For this review, take the finished solid that the model builds, in its own axes (mm). Round coordinates to 2 decimals unless told otherwise and drop trailing zeros. Write each loop counter-clockwise with the first axis right and the second up, starting at its lowest first coordinate (ties: lowest second). Pieces come first, ordered by that corner, then holes. Notation, with made-up numbers: (79.25, 54) -> (100.25, 54) arc R12 cw to (100.25, 58) -> close; hole circle Ø3 at (-5.5, -13). An arc over 180 degrees is marked (long way). Answer as CSV lines item,"result". Start each with the question number.
Item 1: Take a section at A-A on y = 96.5. Give the boundary of the cut face in (x, z).
Item 2: Wall thickness on probe 1 along Y at (x, z) = (1.6, -1.6); probe 2 along X at (y, z) = (72.5, 0): over which ranges is each line inside the solid? List them lowest first. Write a range as from..to.
Item 3: For pin 1 Ø1 at (y, z) = (43.5, 0.5) entering from -X; pin 2 Ø3.5 at (x, z) = (0, 0) entering from -Y; pin 3 Ø0.5 at (y, z) = (3, -2.5) entering from +X, all flat-tipped, find the tip position at first contact; note any pin that passes through.
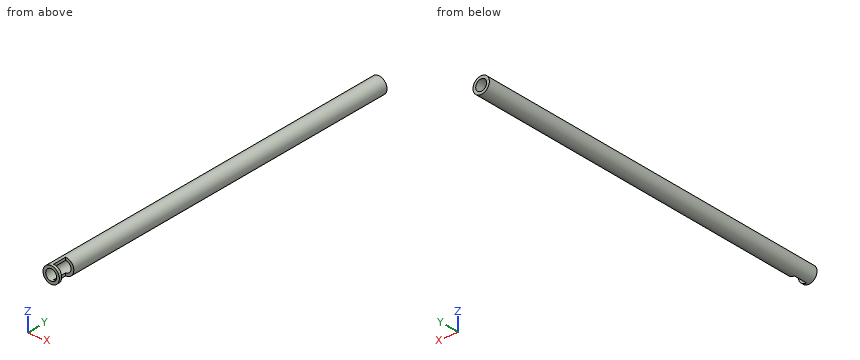
Autodesk Inventor part; units mm, degrees
ref_plane "YZ Plane" through (0, 0, 0) normal (1, 0, 0) x (0, 1, 0)
ref_plane "XZ Plane" through (0, 0, 0) normal (0, 1, 0) x (-1, 0, 0)
ref_plane "XY Plane" through (0, 0, 0) normal (0, 0, 1) x (1, 0, 0)
sketch "Szkic1" plane through (0, 0, 0) normal (0, 1, 0) x (-1, 0, 0)
  circle A0 centre (0, 0) radius 3
  circle A1 centre (0, 0) radius 2
  dimension "d0" = 6
  dimension "d1" = 4
extrude "Wyciągnięcie proste1" add sketch "Szkic1" along normal blind 135
sketch "Szkic2" plane through (0, 0, 0) normal (0, -1, 0) x (1, 0, 0)
  circle A0 centre (0, 0) radius 2
  circle A1 centre (0, 0) radius 3
  dimension "d4" = 6
sketch "Szkic3" plane through (0, 0, 0) normal (0, -1, 0) x (1, 0, 0)
  circle A0 centre (0, 0) radius 3
  line L0 (-0.7678, 2.9001) -> (-0.7678, 1.8467)
  circle A1 centre (0, 0) radius 2
  line L1 (-0.7678, -1.8467) -> (-0.7678, -2.9012)
  line L2 (0.7678, 2.9001) -> (0.7678, 1.8467)
  line L3 (0.7678, -1.8467) -> (0.7678, -2.9001)
  line L4 (-5.8889, 4.1288) -> (-0.7678, 4.1288)
  line L5 (-0.7678, 4.1288) -> (-0.7678, -5.0287)
  line L6 (-0.7678, -5.0287) -> (-5.8889, -5.0287)
  line L7 (-5.8889, -5.0287) -> (-5.8889, 4.1288)
  line L8 (0.0074, 4.1288) -> (6.1006, 4.1288)
  line L9 (6.1006, 4.1288) -> (6.1006, -5.0287)
  line L10 (6.1006, -5.0287) -> (0.0074, -5.0287)
  line L11 (0.0074, -5.0287) -> (0.0074, 4.1288)
  point P0 (-0.7678, -2.9001)
extrude "Wyciągnięcie proste2" cut sketch "Szkic3" against normal blind 5 contours A0 L3 A1 L2 | A0 L11 L8 L9 L10 | L2 A1 L11 A0 | A0 L11 A1 L3 | A1 L11 | A0 L5 L6 L7 L4
extrude "Wyciągnięcie proste3" add sketch "Szkic2" along normal blind 1 contours A0 | A1
sketch "Szkic4" plane through (0, -1, 0) normal (0, -1, 0) x (1, 0, 0)
  circle A0 centre (0, 0) radius 2
  dimension "d9" = 4
extrude "Wyciągnięcie proste4" cut sketch "Szkic4" against normal blind 5
properties part number "rurkadoczujnika"
Output values:
1,outline,"circle Ø6 at (0, 0); hole circle Ø4 at (0, 0)"
2,probe 1,"y = -1..0, 5..135"
2,probe 2,"x = -3..-2, 2..3"
3,pin 1,"stops at x = -3"
3,pin 2,"passes through"
3,pin 3,"stops at x = 0.01"
